Geometry check sheet. Reference: the model listing, model coordinates, mm. Face numbers are marked on the shaded views. A direction names the side the tool comes from. Coordinates: 2 decimals unless noted, no trailing zeros. Loops run counter-clockwise (first coordinate to the right, second up) from the corner with the lowest first, then second, coordinate; pieces in that order, holes last. Notation, with made-up numbers: M 89,-22 L 134,-22 A37 ccw 134,14 Z; hole C 7,-37.75 d9. An arc over 180 degrees is marked long. One line per question, with ' | ' between items. Start each with the question number.
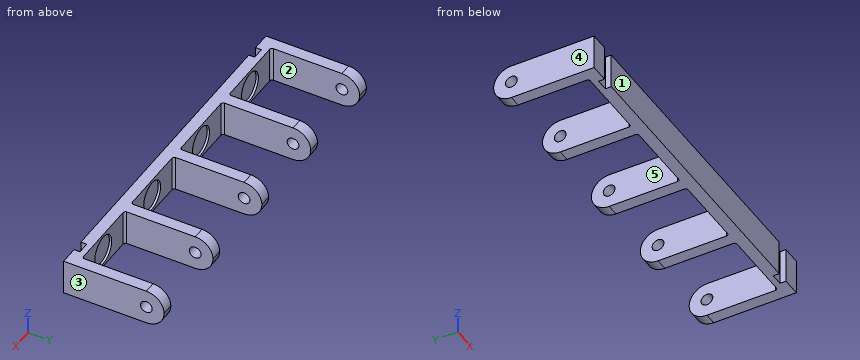
from build123d import *

# Parameters (mm, degrees)
SKETCH1_W            = 300
SKETCH1_H            = 30
BOSS_EXTRUDE1_DEPTH  = 5
SKETCH2_W            = 10
SKETCH2_H            = 30
CUT_EXTRUDE1_DEPTH   = 5
SKETCH3_W            = 10
SKETCH3_H            = 75
BOSS_EXTRUDE2_DEPTH  = 15
FILLET1_R            = 15
SKETCH4_R            = 5
CUT_EXTRUDE2_DEPTH   = 311.845620847
FILLET2_R            = 15
FILLET3_R            = 2
SKETCH5_R            = 12.5
CUT_EXTRUDE3_DEPTH   = 2
LPATTERN1_COUNT      = 3
LPATTERN1_PITCH      = 72.5
LPATTERN1_COUNT_DIR2 = 3
LPATTERN1_PITCH_DIR2 = 72.5


with BuildPart() as part:
    # Sketch1 → Boss-Extrude1 (new, symmetric)
    with BuildSketch(Plane(origin=(0, 0, 0), x_dir=(1, 0, 0), z_dir=(0, 1, 0))):
        Rectangle(SKETCH1_W, SKETCH1_H)
    extrude(amount=BOSS_EXTRUDE1_DEPTH, both=True)

    # Sketch2 → Cut-Extrude1 (cut)
    with BuildSketch(Plane.XZ.offset(5)):
        with Locations((-129.545, 0)):
            Rectangle(SKETCH2_W, SKETCH2_H)
        with Locations((129.545, 0)):
            Rectangle(SKETCH2_W, SKETCH2_H)
    extrude(amount=-CUT_EXTRUDE1_DEPTH, mode=Mode.SUBTRACT)

    # Sketch3 → Boss-Extrude2 (add, symmetric)
    with BuildSketch(Plane.XY):
        with Locations((-145, 42.5)):
            Rectangle(SKETCH3_W, SKETCH3_H)
        with Locations((145, 42.5)):
            Rectangle(SKETCH3_W, SKETCH3_H)
        with Locations((-72.5, 42.5)):
            Rectangle(SKETCH3_W, SKETCH3_H)
        with Locations((72.5, 42.5)):
            Rectangle(SKETCH3_W, SKETCH3_H)
        with Locations((0, 42.5)):
            Rectangle(SKETCH3_W, SKETCH3_H)
    extrude(amount=BOSS_EXTRUDE2_DEPTH, both=True)

    # Fillet1
    fillet1_edges = [part.edges().sort_by_distance(p)[0] for p in [
        (145, 80, -15),
        (145, 80, 15),
        (-145, 80, -15),
        (-145, 80, 15),
    ]]
    fillet(fillet1_edges, radius=FILLET1_R - 0.0001)  # a hair under: the kernel refuses the full size

    # Sketch4 → Cut-Extrude2 (cut, through all)
    with BuildSketch(Plane.ZY.offset(150)):
        with Locations((0, 65)):
            Circle(SKETCH4_R)
    extrude(amount=-CUT_EXTRUDE2_DEPTH, mode=Mode.SUBTRACT)

    # Fillet2
    fillet2_edges = [part.edges().sort_by_distance(p)[0] for p in [
        (72.5, 80, -15),
        (72.5, 80, 15),
        (0, 80, -15),
        (0, 80, 15),
        (-72.5, 80, -15),
        (-72.5, 80, 15),
    ]]
    fillet(fillet2_edges, radius=FILLET2_R - 0.0001)  # a hair under: the kernel refuses the full size

    # Fillet3
    fillet3_edges = [part.edges().sort_by_distance(p)[0] for p in [
        (-140, 5, 0),
        (140, 5, 0),
        (-77.5, 5, 0),
        (-67.5, 5, 0),
        (67.5, 5, 0),
        (77.5, 5, 0),
        (-5, 5, 0),
        (5, 5, 0),
    ]]
    fillet(fillet3_edges, radius=FILLET3_R)

    # Sketch5 → Cut-Extrude3 (cut)
    with BuildSketch(Plane(origin=(0, 5, 0), x_dir=(1, 0, 0), z_dir=(0, 1, 0))):
        with Locations(Location((36.25, 0, 0), (0, 0, 270))):
            Circle(SKETCH5_R)
    cut_extrude3 = extrude(amount=-CUT_EXTRUDE3_DEPTH, mode=Mode.SUBTRACT)

    # LPattern1: Cut-Extrude3 3 × 3
    with Locations(*[Vector(-1, 0, 0) * (i * LPATTERN1_PITCH) + Vector(1, 0, 0) * (j * LPATTERN1_PITCH_DIR2) for i in range(LPATTERN1_COUNT) for j in range(LPATTERN1_COUNT_DIR2) if (i, j) != (0, 0)]):
        add(cut_extrude3, mode=Mode.SUBTRACT)


solid = part.part
1. Thickness scan on line 1 (X direction, y = 71, z = -12); line 2 (X direction, y = 4, z = 0); line 3 (Y direction, x = 145, z = 0). Record the ranges inside material, lowest first.
2. Depth check by flat-ended pin: pin 1 Ø9 at (x, z) = (-102, -2) entering from +Y; pin 2 Ø11 at (x, z) = (-131, 0) entering from -Y. Enter the tip coordinate at first touch or a pass-through.
3. Draft check along X on the marked faces 3, 4 and 5. Enter one of: +X half, -X half, draft (parallel to the pull), parting line (faces both ways), or undercut.
4. Sectioned sample at C-C (x = -113.5). Record the cut outline in (y, z).
5. Sectioned sample at B-B (x = 108.75). Record the cut outline in (y, z), and give its area (3 significant figures).
6. Tool access check on the marked faces 1 and 2. Record the directions out of +Z, -Z, +X, -X, +Y, -Y that give a thin tool (end or side, any length) a straight path to the whole face; none if there is none.
7. Sectioned sample at D-D (y = 74.5). Record the cut outline in (x, z), and give its area (3 significant figures).
8. Sectioned sample at A-A (y = 37). Record the cut outline in (x, z).
Result:
1) line 1: x = -150 to -140, -77.5 to -67.5, -5 to 5, 67.5 to 77.5, 140 to 150 | line 2: x = -150 to -121.25, -96.25 to -48.75, -23.75 to 23.75, 48.75 to 96.25, 121.25 to 150 | line 3: y = -5 to 60, 70 to 80
2) pin 1: stops at y = 3 | pin 2: stops at y = -5
3) face 3: +X half | face 4: -X half | face 5: undercut
4) outline: M -5,-15 L 5,-15 L 5,-11.56 L 3,-11.56 L 3,11.56 L 5,11.56 L 5,15 L -5,15 Z
5) outline: M -5,-15 L 5,-15 L 5,-12.5 L 3,-12.5 L 3,12.5 L 5,12.5 L 5,15 L -5,15 Z | area: 250 mm2
6) face 1: +Z, -Z, +X, -X, -Y | face 2: +Z, -Z, +Y
7) outline: M -150,-11.61 L -140,-11.61 L -140,11.61 L -150,11.61 Z; M -77.5,-11.61 L -67.5,-11.61 L -67.5,11.61 L -77.5,11.61 Z; M -5,-11.61 L 5,-11.61 L 5,11.61 L -5,11.61 Z; M 67.5,-11.61 L 77.5,-11.61 L 77.5,11.61 L 67.5,11.61 Z; M 140,-11.61 L 150,-11.61 L 150,11.61 L 140,11.61 Z | area: 1,160 mm2
8) outline: M -150,-15 L -140,-15 L -140,15 L -150,15 Z; M -77.5,-15 L -67.5,-15 L -67.5,15 L -77.5,15 Z; M -5,-15 L 5,-15 L 5,15 L -5,15 Z; M 67.5,-15 L 77.5,-15 L 77.5,15 L 67.5,15 Z; M 140,-15 L 150,-15 L 150,15 L 140,15 Z
